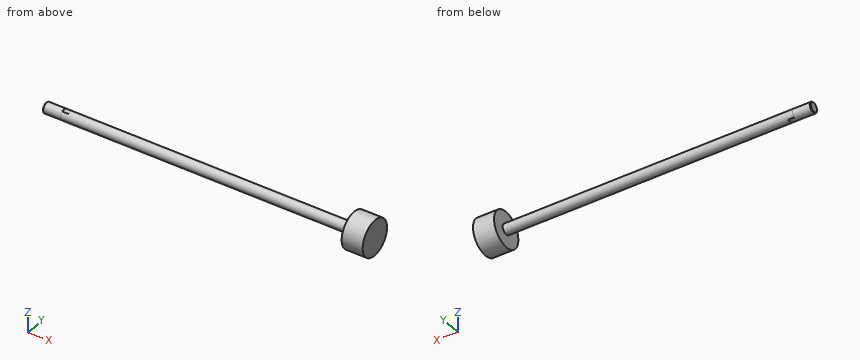
Autodesk Inventor part; units mm, degrees
ref_plane "dia1_XY" through (-6.35, 5.5499, 0) normal (1, 0, 0) x (0, 0, -1)
ref_plane "dia1_YZ" through (-6.35, 5.5499, 0) normal (0, 0, -1) x (0, 1, 0)
ref_plane "dia1_ZX" through (-6.35, 5.5499, 0) normal (0, 1, 0) x (1, 0, 0)
sketch "Sketch_1" plane through (0, 0, 0) normal (0, 0, 1) x (1, 0, 0)
  line L0 (323.977, 0) -> (-6.35, 0)
  line L1 (-6.35, 0) -> (-6.35, 5.5499)
  line L2 (-6.35, 5.5499) -> (301.625, 5.5499)
  line L3 (301.625, 5.5499) -> (301.625, 19.1453)
  line L4 (301.625, 19.1453) -> (323.977, 19.1453)
  line L5 (323.977, 19.1453) -> (323.977, 0)
  line L6 (323.977, 0) -> (-6.35, 0)
revolve "Revolution1" add sketch "Sketch_1" angle 360 about axis through (323.977, 0, 0) along (1, 0, 0)
sketch "Sketch_3" plane through (0, 0, 0) normal (0, 0, 1) x (1, 0, 0)
  line L0 (-6.35, 0) -> (-25.4, 0)
  line L1 (-25.4, 0) -> (-25.4, 4.8006)
  line L2 (-25.4, 4.8006) -> (-24.6443, 5.5563)
  line L3 (-24.6443, 5.5563) -> (-6.35, 5.5563)
  line L4 (-6.35, 5.5563) -> (-6.35, 0)
  line L5 (-6.35, 0) -> (-25.4, 0)
revolve "Revolution2" add sketch "Sketch_3" angle 360 about axis through (-6.35, 0, 0) along (1, 0, 0)
thread "Thread1"
sketch "Sketch_10" plane through (-6.35, 0, 0) normal (1, 0, 0) x (0, 0, -1)
  line L0 (-11.0998, -11.0998) -> (11.0998, -11.0998)
  line L1 (11.0998, -11.0998) -> (11.0998, 11.0998)
  line L2 (11.0998, 11.0998) -> (-11.0998, 11.0998)
  line L3 (-11.0998, 11.0998) -> (-11.0998, -11.0998)
  line L4 (-4.826, -5.5499) -> (4.826, -5.5499)
  line L5 (4.826, -5.5499) -> (4.826, 5.5499)
  line L6 (4.826, 5.5499) -> (-4.826, 5.5499)
  line L7 (-4.826, 5.5499) -> (-4.826, -5.5499)
extrude "Extrusion1" cut sketch "Sketch_10" along normal blind 6.35
ref_plane "dia1_XY" through (-6.35, 5.5499, 0) normal (1, 0, 0) x (0, 0, -1)
ref_plane "dia1_YZ" through (-6.35, 5.5499, 0) normal (0, 0, -1) x (0, 1, 0)
ref_plane "dia1_ZX" through (-6.35, 5.5499, 0) normal (0, 1, 0) x (1, 0, 0)
ref_plane "dia12_XY" through (0, 0, 19.7675) normal (1, 0, 0) x (0, 0, -1)
ref_plane "dia12_YZ" through (0, 0, 19.7675) normal (0, 0, -1) x (0, 1, 0)
ref_plane "dia12_ZX" through (0, 0, 19.7675) normal (0, 1, 0) x (1, 0, 0)
ref_plane "dia2_XY" through (-6.35, -5.5499, 0) normal (1, 0, 0) x (0, 0, -1)
ref_plane "dia2_YZ" through (-6.35, -5.5499, 0) normal (0, 0, -1) x (0, 1, 0)
ref_plane "dia2_ZX" through (-6.35, -5.5499, 0) normal (0, 1, 0) x (1, 0, 0)
ref_plane "dia22_XY" through (0, 0, -19.7675) normal (1, 0, 0) x (0, 0, -1)
ref_plane "dia22_YZ" through (0, 0, -19.7675) normal (0, 0, -1) x (0, 1, 0)
ref_plane "dia22_ZX" through (0, 0, -19.7675) normal (0, 1, 0) x (1, 0, 0)
ref_plane "rl1_XY" through (-25.4, 0, 0) normal (1, 0, 0) x (0, 0, -1)
ref_plane "rl1_YZ" through (-25.4, 0, 0) normal (0, 0, -1) x (0, 1, 0)
ref_plane "rl1_ZX" through (-25.4, 0, 0) normal (0, 1, 0) x (1, 0, 0)
ref_plane "rl2_XY" through (-6.35, 0, 0) normal (1, 0, 0) x (0, 0, -1)
ref_plane "rl2_YZ" through (-6.35, 0, 0) normal (0, 0, -1) x (0, 1, 0)
ref_plane "rl2_ZX" through (-6.35, 0, 0) normal (0, 1, 0) x (1, 0, 0)
ref_plane "rod_cp_XY" through (0, 0, 0) normal (1, 0, 0) x (0, 0, -1)
ref_plane "rod_cp_YZ" through (0, 0, 0) normal (0, 0, -1) x (0, 1, 0)
ref_plane "rod_cp_ZX" through (0, 0, 0) normal (0, 1, 0) x (1, 0, 0)
ref_plane "thd1_XY" through (-25.4, 5.5563, 0) normal (1, 0, 0) x (0, 0, -1)
ref_plane "thd1_YZ" through (-25.4, 5.5563, 0) normal (0, 0, -1) x (0, 1, 0)
ref_plane "thd1_ZX" through (-25.4, 5.5563, 0) normal (0, 1, 0) x (1, 0, 0)
ref_plane "thd2_XY" through (-25.4, -5.5563, 0) normal (1, 0, 0) x (0, 0, -1)
ref_plane "thd2_YZ" through (-25.4, -5.5563, 0) normal (0, 0, -1) x (0, 1, 0)
ref_plane "thd2_ZX" through (-25.4, -5.5563, 0) normal (0, 1, 0) x (1, 0, 0)
ref_plane "to_rod_clevis_XY" through (-30.988, 0, 0) normal (1, 0, 0) x (0, 0, -1)
ref_plane "to_rod_clevis_YZ" through (-30.988, 0, 0) normal (0, 0, -1) x (0, 1, 0)
ref_plane "to_rod_clevis_ZX" through (-30.988, 0, 0) normal (0, 1, 0) x (1, 0, 0)
ref_plane "wf1_XY" through (-6.35, 0, 0) normal (1, 0, 0) x (0, 0, -1)
ref_plane "wf1_YZ" through (-6.35, 0, 0) normal (0, 0, -1) x (0, 1, 0)
ref_plane "wf1_ZX" through (-6.35, 0, 0) normal (0, 1, 0) x (1, 0, 0)
ref_plane "wf2_XY" through (0, 0, 0) normal (1, 0, 0) x (0, 0, -1)
ref_plane "wf2_YZ" through (0, 0, 0) normal (0, 0, -1) x (0, 1, 0)
ref_plane "wf2_ZX" through (0, 0, 0) normal (0, 1, 0) x (1, 0, 0)
ref_plane "wfw1_XY" through (-6.35, 0, -4.826) normal (0, 1, 0) x (1, 0, 0)
ref_plane "wfw1_YZ" through (-6.35, 0, -4.826) normal (1, 0, 0) x (0, 0, -1)
ref_plane "wfw1_ZX" through (-6.35, 0, -4.826) normal (0, 0, -1) x (0, 1, 0)
ref_plane "wfw2_XY" through (-6.35, 0, 4.826) normal (0, 1, 0) x (1, 0, 0)
ref_plane "wfw2_YZ" through (-6.35, 0, 4.826) normal (1, 0, 0) x (0, 0, -1)
ref_plane "wfw2_ZX" through (-6.35, 0, 4.826) normal (0, 0, -1) x (0, 1, 0)
properties part number "C-175-DPEE50_rod" material "Steel, Galvanized"
The listing builds one solid part. Answer for the finished solid, in the listing's coordinates (mm). Coordinates: 2 decimals unless noted, no trailing zeros. Write each loop counter-clockwise with the first axis right and the second up, starting at its lowest first coordinate (ties: lowest second). Pieces come first, ordered by that corner, then holes. Notation, with made-up numbers: (10.5, 11.25) -> (66.5, 11.25) arc R30 ccw to (66.5, 38.25) -> close; hole circle Ø1 at (5.5, 24.5). An arc over 180 degrees is marked (long way). Write each question's results on one line, items separated by ' | '. Start each with the question number.
1) A cutting plane is placed at B-B (x = 122). Determine the outline of the cut face in (y, z).
2) Flat-ended cylindrical pins translate along their axes: pin 1 Ø1 at (y, z) = (6, -3.5) entering from -X (3 decimals); pin 2 Ø6 at (y, z) = (4.5, 6.5) entering from -X; pin 3 Ø1.6 at (x, y) = (-1.5, -0.5) entering from -Z; pin 4 Ø1 at (x, z) = (94, 7) entering from +Y. Find the tip coordinate at first contact, or state that the pin passes through.
3) Straight lines are drawn through the part: probe 1 along X at (y, z) = (-4, -10) (3 decimals); probe 2 along Y at (x, z) = (46, 4); probe 3 along Z at (x, y) = (26, -1). For each, find the intervals that lie inside material, in ascending order.
4) A cutting plane is placed at A-A (z = 0). Determine the outline of the cut face in (x, y) (3 decimals).
5) A cutting plane is placed at C-C (z = 15). Determine the outline of the cut face in (x, y) (3 decimals), then the cut area to 3 significant figures.
Values follow:
1) outline: circle Ø11.1 at (0, 0)
2) pin 1: x = 301.625 | pin 2: x = -25.29 | pin 3: z = -4.83 | pin 4: through
3) probe 1: 301.625 to 323.977 | probe 2: -3.85 to 3.85 | probe 3: -5.46 to 5.46
4) outline: (-25.4, -4.801) -> (-24.644, -5.556) -> (-6.35, -5.556) -> (-6.35, -5.55) -> (301.625, -5.55) -> (301.625, -19.145) -> (323.977, -19.145) -> (323.977, 19.145) -> (301.625, 19.145) -> (301.625, 5.55) -> (-6.35, 5.55) -> (-6.35, 5.556) -> (-24.644, 5.556) -> (-25.4, 4.801) -> close
5) outline: (301.625, -11.897) -> (323.977, -11.897) -> (323.977, 11.897) -> (301.625, 11.897) -> close | area: 532 mm²
